```python
from build123d import *

# Parameters (mm, degrees)
SKETCH1_W           = 40.4
SKETCH1_H           = 20
BOSS_EXTRUDE1_DEPTH = 36.6
SKETCH2_W           = 2.3
SKETCH2_H           = 20
BOSS_EXTRUDE2_DEPTH = 6.5
SKETCH3_R           = 2.2
CUT_EXTRUDE1_DEPTH  = 6.5
BOSS_EXTRUDE4_DEPTH = 2
BOSS_EXTRUDE5_DEPTH = 1.5
SKETCH7_R           = 6.5
BOSS_EXTRUDE6_DEPTH = 1
SKETCH9_R           = 5.25
BOSS_EXTRUDE7_DEPTH = 0.5
SKETCH10_R          = 4.4
BOSS_EXTRUDE8_DEPTH = 4.5
SKETCH11_R          = 10.6
BOSS_EXTRUDE9_DEPTH = 2
SKETCH12_R          = 1.5
SKETCH12_R_2        = 1.264823641
CUT_EXTRUDE2_DEPTH  = 2
CIRPATTERN1_COUNT   = 2


with BuildPart() as part:
    # Sketch1 → Boss-Extrude1 (new body)
    with BuildSketch(Plane.XY):
        Rectangle(SKETCH1_W, SKETCH1_H)
    extrude(amount=BOSS_EXTRUDE1_DEPTH)

    # Sketch2 → Boss-Extrude2 (add)
    with BuildSketch(Plane(origin=(20.2, 0, 0), x_dir=(0, 0, -1), z_dir=(1, 0, 0))):
        with Locations((-29.15, 0)):
            Rectangle(SKETCH2_W, SKETCH2_H)
    boss_extrude2 = extrude(amount=BOSS_EXTRUDE2_DEPTH)

    # Sketch3 → Cut-Extrude1 (cut)
    with BuildSketch(Plane.XY.offset(30.3)):
        with Locations((24.929249083, -5.5)):
            Circle(SKETCH3_R)
        with Locations((24.929249083, 5.5)):
            Circle(SKETCH3_R)
    cut_extrude1 = extrude(amount=-CUT_EXTRUDE1_DEPTH, mode=Mode.SUBTRACT)

    # Mirror1: Boss-Extrude2, Cut-Extrude1 across plane
    add(boss_extrude2.mirror(Plane(origin=(0, 0, 0), x_dir=(0, 0, 1), z_dir=(1, 0, 0))))
    add(cut_extrude1.mirror(Plane(origin=(0, 0, 0), x_dir=(0, 0, 1), z_dir=(1, 0, 0))), mode=Mode.SUBTRACT)

    # Sketch5 → Boss-Extrude4 (add)
    with BuildSketch(Plane.XY.offset(36.6)):
        with BuildLine():
            Line((5.841101056, 9), (-14.2, 9))
            Line((-14.2, 9), (-14.2, 5.100716034))
            Line((-14.2, 5.100716034), (-14.2, -4.399283966))
            Line((-14.2, -4.399283966), (-14.2, -9))
            Line((-14.2, -9), (5.841101056, -9))
            ThreePointArc((5.841101056, -9), (0.2, 0), (5.841101056, 9))
        make_face()
        with BuildLine():
            ThreePointArc((20.2, 0), (15.510885546, 8.473163206), (5.841101056, 9))
            Line((5.841101056, 9), (5.841101056, -9))
            ThreePointArc((5.841101056, -9), (15.510885546, -8.473163206), (20.2, 0))
        make_face()
        with BuildLine():
            Line((5.841101056, -9), (5.841101056, 9))
            ThreePointArc((5.841101056, 9), (0.2, 0), (5.841101056, -9))
        make_face()
        with BuildLine():
            ThreePointArc((20.2, 0), (15.510885546, 8.473163206), (5.841101056, 9))
            Line((5.841101056, 9), (5.841101056, -9))
            ThreePointArc((5.841101056, -9), (15.510885546, -8.473163206), (20.2, 0))
        make_face()
        with BuildLine():
            Line((5.841101056, -9), (5.841101056, 9))
            ThreePointArc((5.841101056, 9), (0.2, 0), (5.841101056, -9))
        make_face()
    extrude(amount=BOSS_EXTRUDE4_DEPTH)

    # Sketch6 → Boss-Extrude5 (add)
    with BuildSketch(Plane.XY.offset(36.6)):
        with BuildLine():
            Line((-14.2, -4.399283966), (-14.2, 5.100716034))
            ThreePointArc((-14.2, 5.100716034), (-16.842653315, 0.350716034), (-14.2, -4.399283966))
        make_face()
    extrude(amount=BOSS_EXTRUDE5_DEPTH)

    # Sketch7 → Boss-Extrude6 (add)
    with BuildSketch(Plane.XY.offset(38.6)):
        with Locations((10.2, 0)):
            Circle(SKETCH7_R)
    extrude(amount=BOSS_EXTRUDE6_DEPTH)

    # Sketch9 → Boss-Extrude7 (add)
    with BuildSketch(Plane.XY.offset(39.6)):
        with Locations((10.2, 0)):
            Circle(SKETCH9_R)
    extrude(amount=BOSS_EXTRUDE7_DEPTH)

    # Sketch10 → Boss-Extrude8 (add)
    with BuildSketch(Plane.XY.offset(40.1)):
        with Locations((10.2, 0)):
            Circle(SKETCH10_R)
    extrude(amount=BOSS_EXTRUDE8_DEPTH)

    # Sketch11 → Boss-Extrude9 (add)
    with BuildSketch(Plane.XY.offset(44.6)):
        with Locations((10.2, 0)):
            Circle(SKETCH11_R)
    extrude(amount=BOSS_EXTRUDE9_DEPTH)

    # Sketch12 → Cut-Extrude2 (cut)
    with BuildSketch(Plane.XY.offset(46.6)):
        with Locations((10.2, 0)):
            Circle(SKETCH12_R)
        with Locations((10.2, -8.1)):
            Circle(SKETCH12_R_2)
    cut_extrude2 = extrude(amount=-CUT_EXTRUDE2_DEPTH, mode=Mode.SUBTRACT)

    # CirPattern1: Cut-Extrude2 ×2 about axis
    cirpattern1_axis = Axis((10.2, 0, 0), (0, 0, 1))
    for i in range(1, CIRPATTERN1_COUNT):
        add(cut_extrude2.rotate(cirpattern1_axis, i * 360 / CIRPATTERN1_COUNT), mode=Mode.SUBTRACT)


solid = part.part
```
Can you work these out from the model? Positions are in its coordinate system, mm. A direction names the side the tool comes from. Coordinates: 2 decimals unless noted, no trailing zeros. Order: outer loops, then holes, each group sorted by start corner. A loop starts at its lowest first (then second) coordinate and runs counter-clockwise, first axis right, second up.
1. If we section it at B-B (z = 12): Please give me the cut outline in (x, y).
2. For faces 1 (the face through (-14.2, 0.1, 38.3)), 2 (the face through (-15, 0, 38.1)), 3 (the face through (15.2, 1.6, 39.8)), which set-ups out of +Z, -Z, +X, -X, +Y, -Y let a thin tool reach every point of the face, with its end or its side?
3. If we section it at A-A (x = -15.5): Please give me the cut outline in (y, z), then the cut area to 3 significant figures.
4. I'm going to push flat-ended pins straight in: pin 1 (2 mm diameter, centred on y = 5.5, z = 38.5, fed in from -X); pin 2 (5.5 mm diameter, centred on x = -24.93, y = -5.5, fed in from +Z); pin 3 (6 mm diameter, centred on x = -20, z = 23.5, fed in from -Y); pin 4 (1.5 mm diameter, centred on x = 11, y = 0.5, fed in from +Z). Where does each tip first touch, or does it pass through?
5. If we section it at C-C (x = -21): Please give me the cut outline in (y, z).
6. I need wall thicknesses on line 1 (Y direction, x = 10.2, z = 46); line 2 (Z direction, x = 15.5, y = -7.25); line 3 (Z direction, x = 20.5, y = 1.75). Which ranges of each line are inside material? Lowest first, please.
7. Thinking about a two-plate mould opening in Y: for faces 4 (the face through (-22.73, -5.42, 29.17)), 5 (the face through (26.7, 8, 29)), 6 (the face through (19.99, -4.06, 45.59)), 7 (the face through (0, -10, 18)), which applies, +Y half, -Y half, draft (parallel to the pull), parting line (faces both ways), or undercut?
Entries:
1. outline: (-20.2, -10) - (20.2, -10) - (20.2, 10) - (-20.2, 10) - close
2. face 1: +Z, -X
2. face 2: +Z, -X, +Y, -Y
2. face 3: none
3. outline: (-10, 0) - (10, 0) - (10, 36.6) - (3.99, 36.6) - (3.99, 38.1) - (-3.28, 38.1) - (-3.28, 36.6) - (-10, 36.6) - close
3. area: 743 mm2
4. pin 1: stops at x = -14.9
4. pin 2: stops at z = 30.3
4. pin 3: stops at y = -10
4. pin 4: stops at z = 46.6
5. outline: (-10, 28) - (10, 28) - (10, 30.3) - (-10, 30.3) - close
6. line 1: y = -10.6 to -9.36, -6.84 to -1.5, 1.5 to 6.84, 9.36 to 10.6
6. line 2: z = 0 to 38.6, 44.6 to 46.6
6. line 3: z = 28 to 30.3, 44.6 to 46.6
7. face 4: undercut
7. face 5: draft
7. face 6: parting line
7. face 7: -Y half
